CAD build for the part. Positions are in the model's coordinates, mm. Round coordinates to 2 decimals unless told otherwise and drop trailing zeros. Order: outer loops, then holes, each group sorted by start corner. A loop starts at its lowest first (then second) coordinate and runs counter-clockwise, first axis right, second up. Notation, with made-up numbers: M 77,-23 L 130,-23 A19 cw 130,0 Z; hole C 3,-39 d5. An arc over 180 degrees is marked long. Put each result on its own line as item: value.
```python
from build123d import *

# Parameters (mm, degrees)
F0_R     = 4.2
F1_DEPTH = 10
F3_D     = 3.6


with BuildPart() as f1:
    # F0 (on Top) → F1 (new body)
    with BuildSketch(Plane.XY):
        Polygon((-31.75, 10.2), (-45.95, 10.2), (-45.95, -10.2), (45.95, -10.2), (45.95, 10.2), align=None)
        with BuildLine():
            ThreePointArc((-27.55, 0), (-34.719848, -2.969848), (-31.75, 4.2))
            ThreePointArc((-31.75, 4.2), (-28.780152, 2.969848), (-27.55, 0))
        make_face(mode=Mode.SUBTRACT)
        with Locations((31.75, 0)):
            Circle(F0_R, mode=Mode.SUBTRACT)
    extrude(amount=F1_DEPTH)

    # F3 (through all)
    with Locations(Plane(origin=(0, 10.2, 0), x_dir=(-1, 0, 0), z_dir=(0, 1, 0))):
        with Locations((-31.75, 5), (-21.75, 5), (21.75, 5), (31.75, 5), (6.75, 5)):
            Hole(F3_D / 2)


solid = f1.part
```
Item 1: Band-saw the part on B-B on y = -5.25. Give the cut face in (x, z), and give its area (3 significant figures).
Answers below:
outline: M -45.95,0 L 45.95,0 L 45.95,10 L -45.95,10 Z; hole C -31.75,5 d3.6; hole C -21.75,5 d3.6; hole C -6.75,5 d3.6; hole C 21.75,5 d3.6; hole C 31.75,5 d3.6
area: 868 mm²
Item 2: Band-saw the part on D-D on x = 31.75. Give the cut face in (y, z).
Answers below:
outline: M -10.2,0 L -4.2,0 L -4.2,3.2 L -10.2,3.2 Z; M -10.2,6.8 L -4.2,6.8 L -4.2,10 L -10.2,10 Z; M 4.2,0 L 10.2,0 L 10.2,3.2 L 4.2,3.2 Z; M 4.2,6.8 L 10.2,6.8 L 10.2,10 L 4.2,10 Z
Item 3: Mould opens along Y. For faces 1 (the flat face through (-1, -10.2, 5)), 2 (the flat face through (1, 10.2, 5)), 3 (the cylindrical face through (-22.14, -0.143, 3.243)), 4 (the cylindrical face through (35.756, 1.262, 4.93)) say: pulls with the +Y half, pulls with the -Y half, needs draft (parallel to the pull), parting line crosses it, or undercut.
Answers below:
face 1: pulls with the -Y half
face 2: pulls with the +Y half
face 3: needs draft
face 4: undercut
Item 4: Band-saw the part on C-C on z = 5. State how many separate pieces and enclosed holes the cut face has, and give its area (3 significant figures).
Answers below:
separate pieces: 6
enclosed holes: 0
area: 1,460 mm²
Item 5: Band-saw the part on A-A on x = -21.75. Give the cut face in (y, z), and give its area (3 significant figures).
Answers below:
outline: M -10.2,0 L 10.2,0 L 10.2,3.2 L -10.2,3.2 Z; M -10.2,6.8 L 10.2,6.8 L 10.2,10 L -10.2,10 Z
area: 131 mm²
Item 6: Probe line 1 along Z through (x, y) = (21.75, 0.25); line 2 along X through (y, z) = (6.5, 5.5); line 3 along X through (y, z) = (-2.25, 6.5). List the from-to ranges inside material, lowest first. Write a range as [from, to].
Answers below:
line 1: [0, 3.2], [6.8, 10]
line 2: [-45.95, -33.48], [-30.02, -23.48], [-20.02, -8.48], [-5.02, 20.02], [23.48, 30.02], [33.48, 45.95]
line 3: [-45.95, -35.3], [-28.2, -22.74], [-20.76, -7.74], [-5.76, 20.76], [22.74, 28.2], [35.3, 45.95]
Item 7: Pin check, flat tip, straight feed: P1, Ø3, axis at x = -31.75, z = 5, coming from the +Y side. Stop position of the tip, or through.
Answers below:
P1: through
